from build123d import *

# Parameters (mm, degrees)
BOSS_EXTRUDE1_DEPTH = 5
BOSS_EXTRUDE3_DEPTH = 50


with BuildPart() as part:
    # Sketch1 → Boss-Extrude1 (new body)
    with BuildSketch(Plane.XY):
        Polygon((0, 0), (0, 37), (9.5, 37), (9.5, 4), (53.5, 4), (53.5, 14), (63, 14), (63, 0), align=None)
    extrude(amount=BOSS_EXTRUDE1_DEPTH)

    # Sketch2 → Boss-Extrude3 (add)
    with BuildSketch(Plane.XY.offset(5)):
        Polygon((0, 37), (14.5, 37), (14.5, 14), (63, 14), (63, 0), (0, 0), align=None)
    extrude(amount=BOSS_EXTRUDE3_DEPTH)


solid = part.part
Design review of the part built by this model. Coordinates are the model's own, in mm. A direction names the side the tool comes from. Round coordinates to 2 decimals unless told otherwise and drop trailing zeros. Write each loop counter-clockwise with the first axis right and the second up, starting at its lowest first coordinate (ties: lowest second). Pieces come first, ordered by that corner, then holes. Notation, with made-up numbers: (-2.75, 21) - (43.25, 21) arc R9 ccw to (43.25, 29) - close; hole circle Ø5 at (-24.75, -22). An arc over 180 degrees is marked (long way). Return JSON: item names as keys, results as strings. Group by question number.
Item 1: For probe 1 along Y at (x, z) = (40.5, 33.5); probe 2 along X at (y, z) = (25, 9.5); probe 3 along Z at (x, y) = (42, 9), list the stretches that pass through material, from the lowest coordinate up. Write a range as [from, to].
Item 2: We need section B-B on y = 12.5. Write out the cut boundary in (x, z).
Item 3: We need section D-D on y = 32. Write out the cut boundary in (x, z), and give its area (4 significant figures).
Item 4: We need section C-C on x = 18. Write out the cut boundary in (y, z).
Item 5: Insertion check: P1, Ø5.5, axis at x = 20.5, z = 2, coming from the +Y side; P2, Ø8, axis at y = 28, z = 21.5, coming from the +X side; P3, Ø14.5, axis at x = 34.5, z = 35, coming from the +Y side; P4, Ø18.5, axis at y = 23, z = 31, coming from the +X side. Each pin has a flat end and moves straight along its axis. Give the tip position at first contact, or say it passes through.
Item 6: We need section A-A on z = 4. Write out the cut boundary in (x, y), and give its area (4 significant figures).
Item 7: Machinability: for faces 1 (the face through (63, 7, 27)), 2 (the face through (31, 4, 2)), 3 (the face through (38, 14, 27)), which of the approach directions +Z, -Z, +X, -X, +Y, -Y give a long, thin tool a straight path to every point of the face, cutting with its end or side? Answer none if there is none.
Item 8: The part is to be moulded in two halves that separate along X. For faces 4 (the face through (14.5, 26, 30)), 5 (the face through (25, 11, 55)), 6 (the face through (53.5, 9, 2)), say which applies: pulls with the +X half, pulls with the -X half, needs draft (parallel to the pull), parting line crosses it, or undercut.
Model answer:
{
 "1": {"probe 1": "y = [0, 14]", "probe 2": "x = [0, 14.5]", "probe 3": "z = [5, 55]"},
 "2": {"outline": "(0, 0) - (9.5, 0) - (9.5, 5) - (53.5, 5) - (53.5, 0) - (63, 0) - (63, 55) - (0, 55) - close"},
 "3": {"outline": "(0, 0) - (9.5, 0) - (9.5, 5) - (14.5, 5) - (14.5, 55) - (0, 55) - close", "area": "772.5 mm²"},
 "4": {"outline": "(0, 0) - (4, 0) - (4, 5) - (14, 5) - (14, 55) - (0, 55) - close"},
 "5": {"P1": "stops at y = 4", "P2": "stops at x = 14.5", "P3": "stops at y = 14", "P4": "stops at x = 63"},
 "6": {"outline": "(0, 0) - (63, 0) - (63, 14) - (53.5, 14) - (53.5, 4) - (9.5, 4) - (9.5, 37) - (0, 37) - close", "area": "660.5 mm²"},
 "7": {"face 1": "+Z, -Z, +X, +Y, -Y", "face 2": "-Z, +Y", "face 3": "+Z, -Z, +X, +Y"},
 "8": {"face 4": "pulls with the +X half", "face 5": "needs draft", "face 6": "undercut"}
}
